from build123d import *

# Parameters (mm, degrees)
F1_DEPTH = 10.668
F3_COUNT = 3
F4_R     = 6.223
F5_DEPTH = 2.54
F6_R     = 5.3975
F7_DEPTH = 25.4


with BuildPart() as f1:
    # F0 (on Top) → F1 (new body)
    with BuildSketch(Plane.XY):
        with BuildLine():
            ThreePointArc((-1.558636, 11.323231), (7.510982, 8.615687), (11.43, 0))
            ThreePointArc((11.43, 0), (7.510982, -8.615687), (-1.558636, -11.323231))
            Line((-1.558636, -11.323231), (25.861818, -15.097641))
            ThreePointArc((25.861818, -15.097641), (12.7, 0), (25.861818, 15.097641))
            Line((25.861818, 15.097641), (-1.558636, 11.323231))
        make_face()
        with BuildLine():
            ThreePointArc((-1.558636, -11.323231), (7.510982, -8.615687), (11.43, 0))
            ThreePointArc((11.43, 0), (7.510982, 8.615687), (-1.558636, 11.323231))
            ThreePointArc((-1.558636, 11.323231), (-11.43, 0), (-1.558636, -11.323231))
        make_face()
        with BuildLine():
            ThreePointArc((43.18, 0), (37.954642, 11.487582), (25.861818, 15.097641))
            ThreePointArc((25.861818, 15.097641), (12.7, 0), (25.861818, -15.097641))
            ThreePointArc((25.861818, -15.097641), (37.954642, -11.487582), (43.18, 0))
        make_face()
        Polygon((40.551639, 0), (34.24582, -10.922), (21.63418, -10.922), (15.328361, 0), (21.63418, 10.922), (34.24582, 10.922), align=None, mode=Mode.SUBTRACT)
    extrude(amount=F1_DEPTH)

    # F3: F1 ×3 about axis
    f3_axis = Axis((0, 0, 10.668), (0, 0, -1))


with BuildPart() as f1_1:
    add(f1.part)
    for i in range(1, F3_COUNT):
        add(f1.part.rotate(f3_axis, i * 360 / F3_COUNT))

    # F4 (on face) → F5 (cut)
    with BuildSketch(Plane(origin=(0, 0, 0), x_dir=(1, 0, 0), z_dir=(0, 0, -1))):
        Circle(F4_R)
    extrude(amount=-F5_DEPTH, mode=Mode.SUBTRACT)

    # F6 (on face) → F7 (cut)
    with BuildSketch(Plane(origin=(0, 0, 2.54), x_dir=(1, 0, 0), z_dir=(0, 0, -1))):
        Circle(F6_R)
    extrude(amount=-F7_DEPTH, mode=Mode.SUBTRACT)


solid = f1_1.part
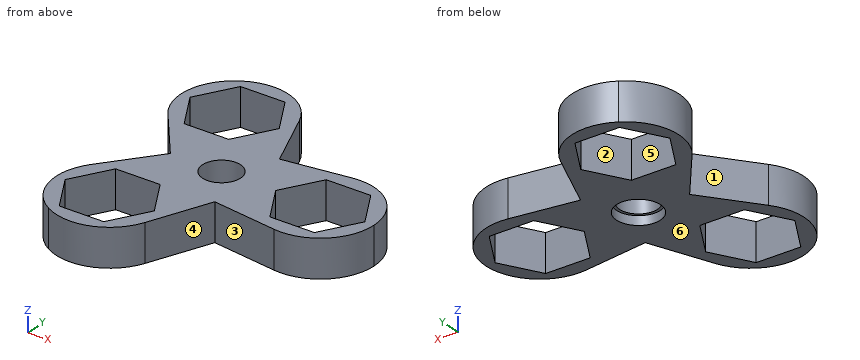
Build history of the part. All positions in model axes, mm. Face numbers are marked on the shaded views. A direction names the side the tool comes from. Coordinates: 2 decimals unless noted, no trailing zeros. Order: outer loops, then holes, each group sorted by start corner. A loop starts at its lowest first (then second) coordinate and runs counter-clockwise, first axis right, second up. Notation, with made-up numbers: (-19.75, -11) - (-3.75, -11) arc R13 ccw to (-3.75, 7) - close; hole circle Ø9 at (-4.75, -39). An arc over 180 degrees is marked (long way). Put each result on its own line as item: value.
1. Saw through at B-B (y = -8.5). Write the cut outline in (x, z), and give its area (3 significant figures).
Answer sheet:
outline: (-21.08, 0) - (20.24, 0) - (20.24, 10.67) - (-21.08, 10.67) - close; (35.64, 0) - (40.59, 0) - (40.59, 10.67) - (35.64, 10.67) - close
area: 493 mm^2
2. Saw through at A-A (x = 22.5). Write the cut outline in (y, z).
Answer sheet:
outline: (-14.63, 0) - (-10.92, 0) - (-10.92, 10.67) - (-14.63, 10.67) - close; (10.92, 0) - (14.63, 0) - (14.63, 10.67) - (10.92, 10.67) - close
3. Pull direction Y, two halves, no side cores. Call the marked faces 4, 5 and 6: pulls with the +Y half, pulls with the -Y half, needs draft (parallel to the pull), parting line crosses it, or undercut.
Answer sheet:
face 4: pulls with the -Y half
face 5: undercut
face 6: needs draft
4. Drop flat-ended pins along their axis: P1, Ø6, axis at x = 11, z = 1.5, coming from the +Y side; P2, Ø5.5, axis at x = 27, z = 7.5, coming from the -Y side; P3, Ø1.5, axis at x = 30, z = 9, coming from the +Y side. Give the stop position or say it passes through.
Answer sheet:
P1: stops at y = 13.46
P2: stops at y = -15.24
P3: stops at y = 15.18
5. Saw through at C-C (y = 4.5). Write the cut outline in (x, z).
Answer sheet:
outline: (-17.97, 0) - (-4.3, 0) - (-4.3, 2.54) - (-2.98, 2.54) - (-2.98, 10.67) - (-17.97, 10.67) - close; (2.98, 2.54) - (4.3, 2.54) - (4.3, 0) - (17.93, 0) - (17.93, 10.67) - (2.98, 10.67) - close; (37.95, 0) - (42.5, 0) - (42.5, 10.67) - (37.95, 10.67) - close
6. Tool access for the marked faces 1, 2 and 3: list every direction of +Z, -Z, +X, -X, +Y, -Y with a clear straight run to the whole face (end or side of a thin tool).
Answer sheet:
face 1: +Z, -Z, -X
face 2: +Z, -Z
face 3: +Z, -Z, -Y
7. Probe line 1 along X through (y, z) = (0, 5.5); line 2 along Y through (x, z) = (-13.5, 6.75); line 3 along X through (y, z) = (0, 0.95). List the from-to ranges inside material, lowest first. Write a range as [from, to].
Answer sheet:
line 1: x = [-14.47, -5.4], [5.4, 15.33], [40.55, 43.18]
line 2: y = [-39.43, -35.12], [-13.27, 13.27], [35.12, 39.43]
line 3: x = [-14.47, -6.22], [6.22, 15.33], [40.55, 43.18]
